```python
from build123d import *

# Parameters (mm, degrees)
F1_DEPTH = 177.8
F2_R     = 50.8
F4_DEPTH = 1676.4


with BuildPart() as f1:
    # F0 (on Right) → F1 (new body)
    with BuildSketch(Plane.YZ):
        with BuildLine():
            add(Edge.make_bspline(
                [(757.3677897453, 430.6074678898), (773.7689614296, 408.6542957115), (839.0123964927, 368.5044864347), (839.0123964927, 295.3796386719)],
                knots=[0, 0, 0, 0, 157.9633109488, 157.9633109488, 157.9633109488, 157.9633109488], degree=3))
            Line((757.3677897453, 430.6074678898), (-839.0123964927, 430.6074678898))
            Line((-839.0123964927, 430.6074678898), (-839.0123964927, -430.6074678898))
            Line((-839.0123964927, -430.6074678898), (-839.0123964927, -456.0074678898))
            Line((-839.0123964927, -456.0074678898), (-601.4769821503, -456.0074678898))
            add(Edge.make_bspline(
                [(-601.4769821503, -456.0074678898), (-562.1427297592, -455.1187157631), (-541.7929887772, -443.0595934391), (-536.967917018, -406.0792799859)],
                knots=[0, 0, 0, 0, 81.5735461508, 81.5735461508, 81.5735461508, 81.5735461508], degree=3))
            ThreePointArc((-536.967917018, -406.0792799859), (-258.1997910033, -122.9745139814), (63.6125510645, -355.9912367912))
            ThreePointArc((63.6125510645, -355.9912367912), (64.9345219834, -361.7820753858), (66.1433977712, -367.5975751983))
            add(Edge.make_bspline(
                [(66.1433977712, -367.5975751983), (79.3549297873, -412.2478035768), (127.0050581979, -426.72), (163.3523256442, -426.72)],
                knots=[9.2699794157, 9.2699794157, 9.2699794157, 9.2699794157, 122.2725667444, 122.2725667444, 122.2725667444, 122.2725667444], degree=3))
            Line((163.3523256442, -426.72), (737.405538559, -426.72))
            add(Edge.make_bspline(
                [(737.405538559, -426.72), (796.8827855437, -426.72), (828.529104676, -398.0098366737), (839.0123964927, -323.7623274326)],
                knots=[0, 0, 0, 0, 144.6521203428, 144.6521203428, 144.6521203428, 144.6521203428], degree=3))
            Line((839.0123964927, -323.7623274326), (839.0123964927, 295.3796386719))
        make_face()
    extrude(amount=F1_DEPTH)

    # F2
    f2_edges = [f1.edges().sort_by_distance(p)[0] for p in [
        (177.8, 839.012396, -14.191344),
    ]]
    fillet(f2_edges, radius=F2_R)


with BuildPart() as f4:
    # F3 (on face) → F4 (new body)
    with BuildSketch(Plane(origin=(0, 839.0123964927, 0), x_dir=(-1, 0, 0), z_dir=(0, 1, 0))):
        with BuildLine():
            Line((342.2788688957, 421.2450157881), (228.425770998, 421.2450157881))
            add(Edge.make_bspline(
                [(228.425770998, 421.2450157881), (200.5402892828, 342.3034548759), (157.4753234207, 355.173677206), (146.9143778086, 274.7348248959)],
                knots=[0, 0, 0, 0, 167.6584124193, 167.6584124193, 167.6584124193, 167.6584124193], degree=3))
            Line((146.9143778086, 274.7348248959), (162.6101124127, -277.5926335351))
            add(Edge.make_bspline(
                [(162.6101124127, -277.5926335351), (170.5097854137, -353.7607491016), (183.3800077438, -391.2988901138), (201.612830162, -442.3549842119)],
                knots=[0, 0, 0, 0, 169.3158119976, 169.3158119976, 169.3158119976, 169.3158119976], degree=3))
            Line((201.612830162, -442.3549842119), (342.2788688957, -442.3549842119))
            Line((342.2788688957, -442.3549842119), (342.2788688957, 421.2450157881))
        make_face()
    extrude(amount=-F4_DEPTH)


solid = f4.part
```
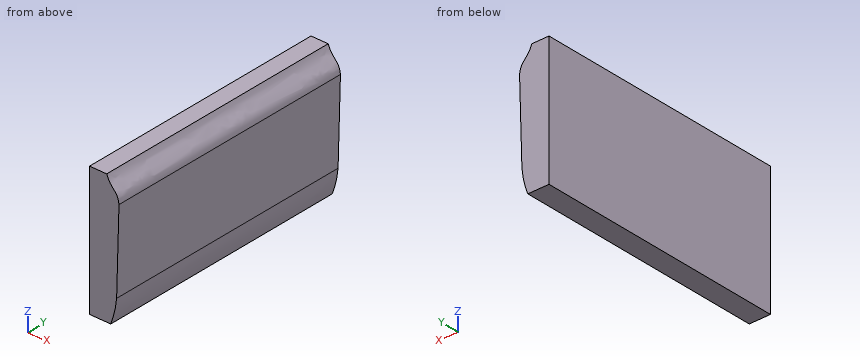
Geometry: final body of the model. Coordinates: model frame, mm. Round coordinates to 2 decimals unless told otherwise and drop trailing zeros. Write each loop counter-clockwise with the first axis right and the second up, starting at its lowest first coordinate (ties: lowest second). Pieces come first, ordered by that corner, then holes.
Item 1: Section query A-A (z = -242.5). Return loops of the section in (x, y), plus the area to 3 significant figures.
Item 2: Pin query (flat end, axial travel): P1, Ø1, axis at y = -207, z = -228, coming from the +X side; P2, Ø1, axis at y = -366, z = -124, coming from the +X side; P3, Ø1.5, axis at y = -336, z = -349.5, coming from the +X side. Return the tip coordinate at first contact, or that it passes through.
Item 3: Material intervals for L1, parallel to X at y = -51.5, z = -326.5; L2, parallel to X at y = -752, z = 176; L3, parallel to Z at x = -215.5, y = 505.5, sorted ascending.
Completed:
1. outline: (-342.28, -837.39) - (-161.61, -837.39) - (-161.61, 839.01) - (-342.28, 839.01) - close
1. area: 303,000 mm2
2. P1: stops at x = -161.19
2. P2: stops at x = -158.23
2. P3: stops at x = -173.4
3. L1: x = -342.28 to -169.17
3. L2: x = -342.28 to -149.72
3. L3: z = -442.35 to 392.16
